Build history of the part. All positions in model axes, mm. A direction names the side the tool comes from. Round coordinates to 2 decimals unless told otherwise and drop trailing zeros. Loops run counter-clockwise (first coordinate to the right, second up) from the corner with the lowest first, then second, coordinate; pieces in that order, holes last. Notation, with made-up numbers: (-2, -8) -> (42, -8) arc R24 cw to (42, 16) -> close; hole circle Ø5 at (-32.75, 89.25). An arc over 180 degrees is marked (long way). Put each result on its own line as item: value. Start each with the question number.
Item 1: Cut at D-D, the plane y = -9.5. List the corners of the cut face in (x, z).
Item 2: Drill centre lines: probe 1 along Y at (x, z) = (-7.5, 4); probe 2 along Z at (x, y) = (-3.5, -2.5). Where is each one in solid material? Low to high. Write a range as [from, to].
Item 3: Tool access for faces 1 (the flat face through (0, -0.23, -3)), 2 (the flat face through (3.8, -4, -38)), 3 (the flat face through (-3.8, -5, -39)): list every direction of +Z, -Z, +X, -X, +Y, -Y with a clear straight run to the whole face (end or side of a thin tool).
Item 4: Flat gauge pins, fed straight in: pin 1 Ø10 at (x, y) = (-4.5, -11) entering from -Z; pin 2 Ø8 at (x, y) = (-6.5, -11.5) entering from +Z; pin 3 Ø6 at (y, z) = (-3, -30) entering from +X; pin 4 Ø5 at (y, z) = (-4, -28) entering from -X. Where does each tip first touch, or does it go through?
```python
from build123d import *

# Parameters (mm, degrees)
BOSS_EXTRUDE1_DEPTH = 0.23
SKETCH2_W           = 38.1
SKETCH2_H           = 38.1
CUT_EXTRUDE1_DEPTH  = 0.01
BOSS_EXTRUDE2_DEPTH = 3.8
CUT_EXTRUDE2_DEPTH  = 3.8


with BuildPart() as part:
    # Sketch1 → Boss-Extrude1 (new body, symmetric)
    with BuildSketch(Plane(origin=(0, 0, 0), x_dir=(1, 0, 0), z_dir=(0, 1, 0))):
        Polygon((3.8, 21.85), (21.85, 21.85), (21.85, -21.85), (-21.85, -21.85), (-21.85, 21.85), (-3.8, 21.85), (-3.8, 61.95), (3.8, 61.95), align=None)
    extrude(amount=BOSS_EXTRUDE1_DEPTH, both=True)

    # Sketch2 → Cut-Extrude1 (cut)
    with BuildSketch(Plane(origin=(0, 0.23, 0), x_dir=(1, 0, 0), z_dir=(0, 1, 0))):
        Rectangle(SKETCH2_W, SKETCH2_H)
    extrude(amount=-CUT_EXTRUDE1_DEPTH, mode=Mode.SUBTRACT)

    # Sketch3 → Boss-Extrude2 (add, symmetric)
    with BuildSketch(Plane(origin=(0, 0, 0), x_dir=(0, 0, -1), z_dir=(1, 0, 0))):
        with BuildLine():
            Line((26.315584349, 0.23), (26.315584349, -0.23))
            ThreePointArc((26.315584349, -0.23), (39.394431992, -5.647436074), (44.811868066, -18.726283717))
            Line((44.811868066, -18.726283717), (45.271868066, -18.726283717))
            ThreePointArc((45.271868066, -18.726283717), (39.719701111, -5.322166955), (26.315584349, 0.23))
        make_face()
    extrude(amount=BOSS_EXTRUDE2_DEPTH, both=True)

    # Sketch4 → Cut-Extrude2 (cut, symmetric)
    with BuildSketch(Plane(origin=(0, 0, 0), x_dir=(0, 0, -1), z_dir=(1, 0, 0))):
        with BuildLine():
            Line((30.466268753, -0.23), (61.95, -0.23))
            Line((61.95, -0.23), (61.95, 0.23))
            Line((61.95, 0.23), (26.315584349, 0.23))
            ThreePointArc((26.315584349, 0.23), (28.403632542, 0.114649039), (30.466268753, -0.23))
        make_face()
    extrude(amount=CUT_EXTRUDE2_DEPTH, both=True, mode=Mode.SUBTRACT)


solid = part.part
```
Reply:
1. outline: (-3.8, -42.88) -> (3.8, -42.88) -> (3.8, -42.35) -> (-3.8, -42.35) -> close
2. probe 1: y = [-0.23, 0.22]
2. probe 2: z = [-36.12, -35.19]
3. face 1: +Z, +X, -X, -Y
3. face 2: -Z, +X, +Y, -Y
3. face 3: -Z, -X, +Y, -Y
4. pin 1: stops at z = -45.07
4. pin 2: stops at z = -41.76
4. pin 3: stops at x = 3.8
4. pin 4: passes through
